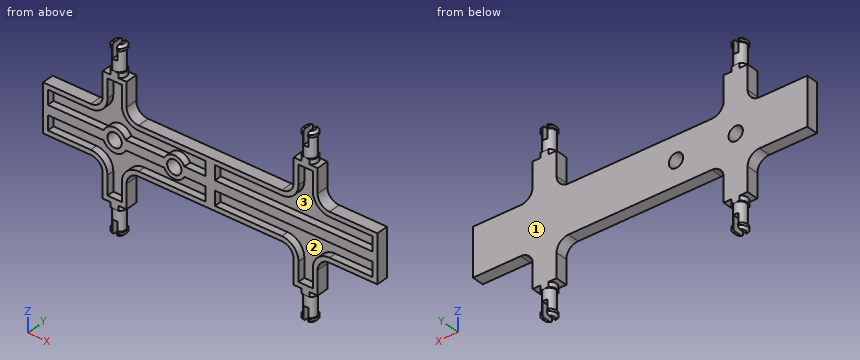
from build123d import *

# Parameters (mm, degrees)
F1_DEPTH  = 2.5
F2_T      = -2
F5_SIZE   = 1
F6_W      = 75.1674278747
F6_H      = 5
F7_DEPTH  = 37.501
F8_W      = 2
F8_H      = 10.0000095664
F9_DEPTH  = 6
F12_R     = 5
F12_R_2   = 4.6528346036
F13_DEPTH = 5
F15_D     = 6


with BuildPart() as f1:
    # F0 (on Front) → F1 (new body, symmetric)
    with BuildSketch(Plane.XZ):
        with BuildLine():
            Line((0, 10), (0, 0))
            Line((0, 0), (70, 0))
            Line((70, 0), (70, 10))
            Line((70, 10), (50, 10))
            ThreePointArc((50, 10), (46.4644660941, 11.4644660941), (45, 15))
            Line((45, 15), (45, 25))
            Line((45, 25), (35, 25))
            Line((35, 25), (35, 15))
            ThreePointArc((35, 15), (33.5355339059, 11.4644660941), (30, 10))
            Line((30, 10), (0, 10))
        make_face()
    extrude(amount=F1_DEPTH, both=True)

    # F2
    f2_openings = [f1.faces().sort_by_distance(p)[0] for p in [
        (35.933685, -2.5, 7.254637),
    ]]
    offset(amount=F2_T, openings=f2_openings)

    # F3 (on Front) → F4 (revolve)
    with BuildSketch(Plane.XZ):
        Polygon((40, 37.5), (37, 37.5), (37, 35.5), (37.5, 35.5), (37.5, 27), (37, 27), (37, 25), (40, 25), align=None)
    revolve(axis=Axis((40, 0, 31.25), (0, 0, -1)))

    # F5
    f5_edges = [f1.edges().sort_by_distance(p)[0] for p in [
        (43, 0, 37.5),
    ]]
    chamfer(f5_edges, length=F5_SIZE)

    # F6 (on face) → F7 (intersect, through all)
    with BuildSketch(Plane.XY.offset(37.5)):
        with Locations((34.6237062477, 0)):
            Rectangle(F6_W, F6_H)
    extrude(amount=-F7_DEPTH, mode=Mode.INTERSECT)

    # F8 (on face) → F9 (cut)
    with BuildSketch(Plane.XY.offset(37.5)):
        with Locations((40, 0.1014110167)):
            Rectangle(F8_W, F8_H)
    extrude(amount=-F9_DEPTH, mode=Mode.SUBTRACT)

    # F10: F1 across plane


with BuildPart() as f1_1:
    add(f1.part)
    add(f1.part.mirror(Plane.XY))

    # F11: F1 across plane


with BuildPart() as f1_2:
    add(f1_1.part)
    add(f1_1.part.mirror(Plane.YZ))

    # F12 (on face) → F13 (join, through all)
    with BuildSketch(Plane.XZ.offset(2.5)):
        with Locations((-40, 0)):
            Circle(F12_R)
        with Locations((-15, 0)):
            Circle(F12_R_2)
    extrude(amount=-F13_DEPTH)

    # F15 (through all)
    with Locations(Plane.XZ.offset(2.5)):
        with Locations((-40, 0), (-15, 0)):
            Hole(F15_D / 2)


solid = f1_2.part
The model under review builds one solid part; all positions refer to its coordinate system, in mm. Face numbers are marked on the shaded views. Round coordinates to 2 decimals unless told otherwise and drop trailing zeros. Write each loop counter-clockwise with the first axis right and the second up, starting at its lowest first coordinate (ties: lowest second). Pieces come first, ordered by that corner, then holes. Notation, with made-up numbers: M 28,44 L 85,44 A21 ccw 85,64 Z; hole C 20.5,-36 d11. An arc over 180 degrees is marked long. Use a Markdown table: item, result. Add a question column.
Q1. We need section A-A, the plane z = -21. State the section outline as (x, y) points.
Q2. Insertion check: pin 1 (2.5 mm diameter, centred on x = -60, y = -1, fed in from -Z); pin 2 (3 mm diameter, centred on x = -2, y = 0.5, fed in from +Z); pin 3 (1.5 mm diameter, centred on y = -1, z = 34, fed in from +X); pin 4 (8 mm diameter, centred on x = 23.5, z = 4.5, fed in from -Y). Each pin has a flat end and moves straight along its axis. Give the tip position at first contact, or say it passes through.
Q3. The part is to be moulded in two halves that separate along X. For the marked faces 1, 2 and 3, say which applies: pulls with the +X half, pulls with the -X half, needs draft (parallel to the pull), parting line crosses it, or undercut.
Q4. We need section D-D, the plane x = -33. State the section outline as (y, z) points.
Q5. We need section C-C, the plane z = 0. State the section outline as (x, y) points, plus the area to 3 significant figures.
Q6. We need section B-B, the plane x = -15. State the section outline as (y, z) points.
Q7. To check wall thickness, follow line 1 (Z direction, x = -15, y = 0.4); line 2 (X direction, y = -0.9, z = -18); line 3 (X direction, y = -1.25, z = 6). State the ranges of each line that lie inside material, in increasing order.
Findings below:
| question | item | result |
|---|---|---|
| 1 | outline | M -45,-2.5 L -43,-2.5 L -43,0.5 L -37,0.5 L -37,-2.5 L -35,-2.5 L -35,2.5 L -45,2.5 Z; M 35,-2.5 L 37,-2.5 L 37,0.5 L 43,0.5 L 43,-2.5 L 45,-2.5 L 45,2.5 L 35,2.5 Z |
| 2 | pin 1 | stops at z = -10 |
| 2 | pin 2 | stops at z = 10 |
| 2 | pin 3 | stops at x = 42.49 |
| 2 | pin 4 | stops at y = -2.5 |
| 3 | face 1 | needs draft |
| 3 | face 2 | undercut |
| 3 | face 3 | undercut |
| 4 | outline | M -2.5,-11 L 2.5,-11 L 2.5,11 L -2.5,11 L -2.5,8.68 L 0.5,8.68 L 0.5,2 L -2.5,2 L -2.5,-2 L 0.5,-2 L 0.5,-8.68 L -2.5,-8.68 Z |
| 5 | outline | M -70,-2.5 L -43,-2.5 L -43,2.5 L -70,2.5 Z; M -37,-2.5 L -18,-2.5 L -18,2.5 L -37,2.5 Z; M -12,-2.5 L 70,-2.5 L 70,2.5 L -12,2.5 Z |
| 5 | area | 640 mm² |
| 6 | outline | M -2.5,-10 L 2.5,-10 L 2.5,-3 L -2.5,-3 L -2.5,-4.65 L 0.5,-4.65 L 0.5,-8 L -2.5,-8 Z; M -2.5,3 L 2.5,3 L 2.5,10 L -2.5,10 L -2.5,8 L 0.5,8 L 0.5,4.65 L -2.5,4.65 Z |
| 7 | line 1 | z = -10 to -8, -4.65 to -3, 3 to 4.65, 8 to 10 |
| 7 | line 2 | x = -45 to -43, -37 to -35, 35 to 37, 43 to 45 |
| 7 | line 3 | x = -70 to -68, -2 to 2, 68 to 70 |
